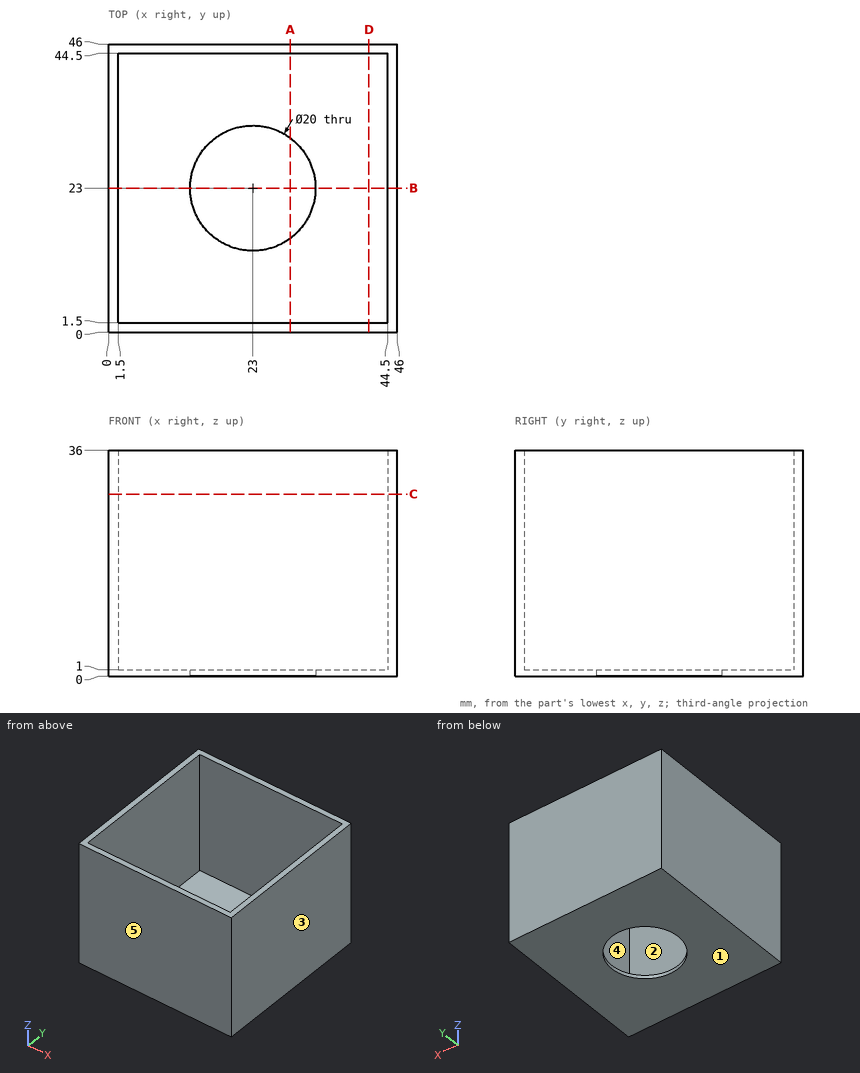
Can you work these out from the drawing? Everything is in mm from the part's minimum corner. A direction names the side the tool comes from. Round coordinates to 2 decimals unless told otherwise and drop trailing zeros. Write each loop counter-clockwise with the first axis right and the second up, starting at its lowest first coordinate (ties: lowest second). Pieces come first, ordered by that corner, then holes. Notation, with made-up numbers: (-12, 3.5) - (25, 3.5) arc R27 ccw to (25, 34.5) - close; hole circle Ø6 at (23.25, 82.25). An arc over 180 degrees is marked (long way). Put each result on its own line as item: value. Start each with the question number.
(1) I need wall thicknesses on probe 1 along Y at (x, z) = (37, 28); probe 2 along Y at (x, z) = (23, 0.2). Which ranges of each line are inside material? Lowest first, please.
(2) I want a section at A-A, the plane x = 29. Please give me the cut outline in (y, z).
(3) Will this pin go through, and if not, where does the flat tip stop? pin 1 (1.5 mm diameter, centred on x = 36, y = 29, fed in from -Z).
(4) For the marked faces 1 and 2, which set-ups out of +Z, -Z, +X, -X, +Y, -Y let a thin tool reach every point of the face, with its end or its side?
(5) Thinking about a two-plate mould opening in Y: for the marked faces 3, 4 and 5, which applies, released by +Y, released by -Y, zero draft, split by the parting line, or undercut?
(6) I want a section at C-C, the plane z = 29. Please give me the cut outline in (x, y), plus the area to 3 significant figures.
(7) I want a section at D-D, the plane x = 41.5. Please give me the cut outline in (y, z).
(8) I want a section at B-B, the plane y = 23. Please give me the cut outline in (x, z), plus the area to 3 significant figures.
Here are the results:
1. probe 1: y = 0 to 1.5, 44.5 to 46
1. probe 2: y = 0 to 13, 33 to 46
2. outline: (0, 0) - (15, 0) - (15, 1) - (1.5, 1) - (1.5, 36) - (0, 36) - close; (31, 0) - (46, 0) - (46, 36) - (44.5, 36) - (44.5, 1) - (31, 1) - close
3. pin 1: stops at z = 0
4. face 1: -Z, +X, -X, +Y, -Y
4. face 2: +Z
5. face 3: zero draft
5. face 4: undercut
5. face 5: released by -Y
6. outline: (0, 0) - (46, 0) - (46, 46) - (0, 46) - close; hole (1.5, 1.5) - (44.5, 1.5) - (44.5, 44.5) - (1.5, 44.5) - close
6. area: 267 mm^2
7. outline: (0, 0) - (46, 0) - (46, 36) - (44.5, 36) - (44.5, 1) - (1.5, 1) - (1.5, 36) - (0, 36) - close
8. outline: (0, 0) - (13, 0) - (13, 1) - (1.5, 1) - (1.5, 36) - (0, 36) - close; (33, 0) - (46, 0) - (46, 36) - (44.5, 36) - (44.5, 1) - (33, 1) - close
8. area: 131 mm^2
